Geometry: see drawing. Coordinates: mm, zero at the bounding-box minimum. A direction names the side the tool comes from. Coordinates: 2 decimals unless noted, no trailing zeros. Order: outer loops, then holes, each group sorted by start corner. A loop starts at its lowest first (then second) coordinate and runs counter-clockwise, first axis right, second up.
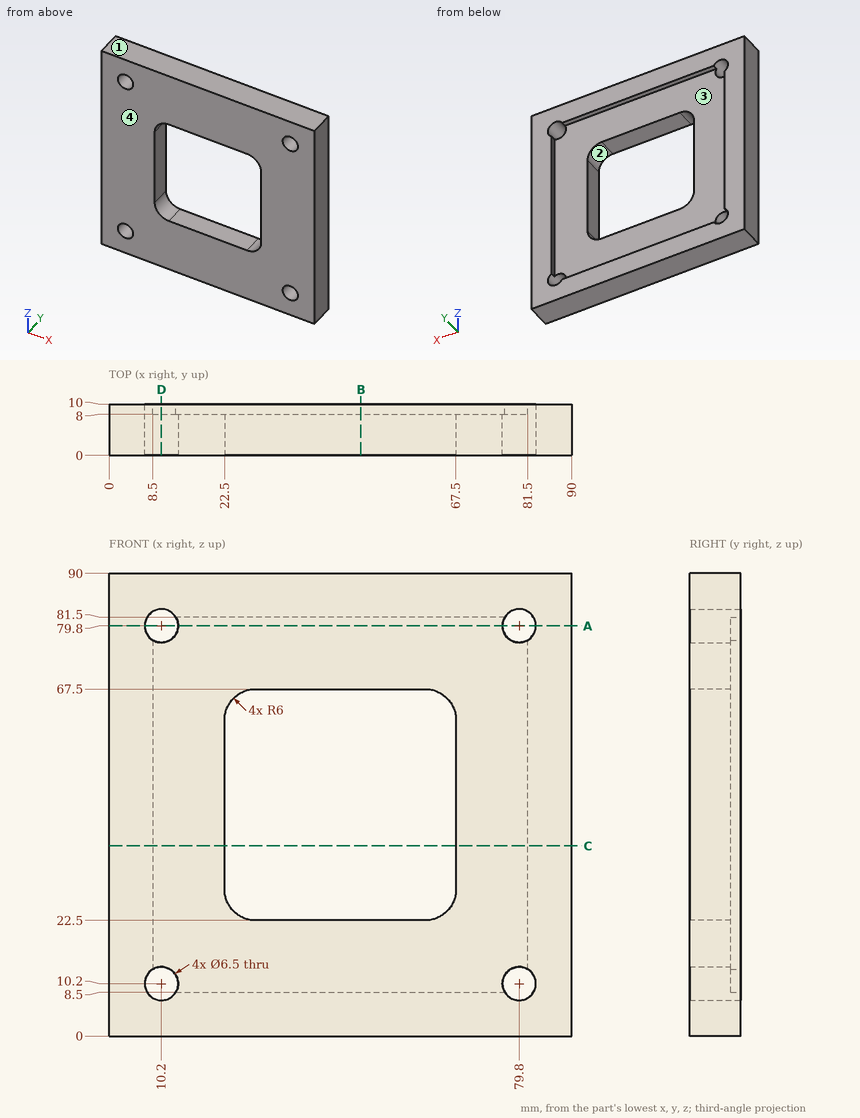
Item 1: Cut plane B-B on x = 49. Return loops of the section in (y, z), then the cut area to 3 significant figures.
Response values:
outline: (0, 0) - (10, 0) - (10, 8.5) - (8, 8.5) - (8, 22.5) - (0, 22.5) - close; (0, 67.5) - (8, 67.5) - (8, 81.5) - (10, 81.5) - (10, 90) - (0, 90) - close
area: 394 mm2
Item 2: Access query for the marked faces 1 and 2. Directions: +Z, -Z, +X, -X, +Y, -Y. A direction counts if a zero-diameter tool reaches every point of the face in a straight line with its end or side. Return the directions, or none.
Response values:
face 1: +Z, +X, -X, +Y, -Y
face 2: +Y, -Y
Item 3: Cut plane A-A on z = 79.8. Return loops of the section in (x, y).
Response values:
outline: (0, 0) - (6.95, 0) - (6.95, 10) - (0, 10) - close; (13.45, 0) - (76.55, 0) - (76.55, 8) - (13.45, 8) - close; (83.05, 0) - (90, 0) - (90, 10) - (83.05, 10) - close
Item 4: Cut plane C-C on z = 37. Return loops of the section in (x, y), then the cut area to 3 significant figures.
Response values:
outline: (0, 0) - (22.5, 0) - (22.5, 8) - (8.5, 8) - (8.5, 10) - (0, 10) - close; (67.5, 0) - (90, 0) - (90, 10) - (81.5, 10) - (81.5, 8) - (67.5, 8) - close
area: 394 mm2
Item 5: Pin query (flat end, axial travel): pin 1 Ø22 at (x, z) = (35.5, 60.5) entering from +Y. Return the tip coordinate at first contact, or that it passes through.
Response values:
pin 1: stops at y = 8
Item 6: Draft query along X for the marked faces 3 and 4. Return one class per face: pulls with the +X half, pulls with the -X half, needs draft (parallel to the pull), parting line crosses it, or undercut.
Response values:
face 3: undercut
face 4: needs draft
Item 7: Cut plane D-D on x = 10.2. Return loops of the section in (y, z), then the cut area to 3 significant figures.
Response values:
outline: (0, 0) - (10, 0) - (10, 6.95) - (0, 6.95) - close; (0, 13.45) - (8, 13.45) - (8, 76.55) - (0, 76.55) - close; (0, 83.05) - (10, 83.05) - (10, 90) - (0, 90) - close
area: 644 mm2
Item 8: Ray query, probe 1 along Z at (x, y) = (10.2, 6); probe 2 along Z at (x, y) = (75, 9.75). Return the intervals inside material, ascending.
Response values:
probe 1: z = 0 to 6.95, 13.45 to 76.55, 83.05 to 90
probe 2: z = 0 to 8.5, 81.5 to 90
